Verification items for the finished model (mm, model axes). A direction names the side the tool comes from. Coordinates: 2 decimals unless noted, no trailing zeros. Write each loop counter-clockwise with the first axis right and the second up, starting at its lowest first coordinate (ties: lowest second). Pieces come first, ordered by that corner, then holes. Notation, with made-up numbers: (-15, 71.25) - (32, 71.25) arc R18 cw to (32, 91.25) - close; hole circle Ø6 at (40.25, -4). An arc over 180 degrees is marked (long way). Use one line per item in the form item = value. Start each with the question number.
(1) Sectioned sample at A-A (y = 16). Record the cut outline in (x, z) (3 decimals), and give its area (3 significant figures).
(2) Sectioned sample at B-B (x = 40). Record the cut outline in (y, z).
(3) Material ranges on line 1 (Y direction, x = 3.25, z = 7.75); line 2 (X direction, y = 30.5, z = 9.5); line 3 (Y direction, x = 31.5, z = 28.5), recorded low to high. Write a range as [from, to].
(4) Gauge pin test, flat ends, axial feed: pin 1 Ø12 at (x, z) = (56.5, 8) entering from +Y (3 decimals); pin 2 Ø4 at (x, z) = (74, 4) entering from +Y; pin 3 Ø8 at (y, z) = (30, 25.5) entering from +X. Record the tip position at first contact, or that the pin passes through.
(5) Mould release check, pull along Z, two halves, no side actions. Record for faces 4 (the flat face through (109, 4, 19)), 5 (the cylindrical face through (114.5, 48.1, 28.8)), 6 (the conical face through (3.215, 59.769, 3.142)): released by +Z, released by -Z, zero draft, split by the parting line, or undercut.
(6) Tool access check on faces 1 (the flat face through (27, 83, 16)), 2 (the flat face through (0, 60, 9)), 3 (the cylindrical face through (114.54, 16.24, 18.97)). Record the directions out of +Z, -Z, +X, -X, +Y, -Y that give a thin tool (end or side, any length) a straight path to the whole face; none if there is none.
(7) Sectioned sample at D-D (y = 39). Record the cut outline in (x, z).
(8) Sectioned sample at C-C (z = 0). Record the cut outline in (x, y).
from build123d import *

# Parameters (mm, degrees)
PAD_DEPTH       = 38
POCKET_DEPTH    = 33
SKETCH015_W     = 6
SKETCH015_H     = 6
PAD006_DEPTH    = 15.5
SKETCH018_W     = 36
SKETCH018_H     = 36
PAD008_DEPTH    = 3.5
POCKET008_DEPTH = 8
SKETCH025_R     = 1.7
HOLE_DEPTH      = 12
HOLE_TIPS_R     = 1.7
SKETCH026_R     = 1.7
HOLE003_DEPTH   = 25
HOLE003_TIPS_R  = 1.7
POCKET009_DEPTH = 1


with BuildPart() as part:
    # Sketch → Pad (new body)
    with BuildSketch(Plane.XY):
        Polygon((-8, -2), (117, -2), (117, 98), (82, 98), (62, 83), (-8, 83), align=None)
    extrude(amount=PAD_DEPTH)

    # Sketch001 (on Face8 of Pad) → Pocket (cut)
    with BuildSketch(Plane.XY.offset(38)):
        Polygon((-3, 75), (-3, 6), (0, 6), (0, 3), (109, 3), (109, 6), (112, 6), (112, 90), (109, 90), (109, 93), (83, 93), (63, 78), (0, 78), (0, 75), align=None)
    extrude(amount=-POCKET_DEPTH, mode=Mode.SUBTRACT)

    # Sketch015 → Pad006 (join)
    with BuildSketch(Plane.XY.offset(3)):
        with Locations((3, 60)):
            Rectangle(SKETCH015_W, SKETCH015_H)
        with Locations((87, 60)):
            Rectangle(SKETCH015_W, SKETCH015_H)
        with Locations((3, 6)):
            Rectangle(SKETCH015_W, SKETCH015_H)
        with Locations((87, 6)):
            Rectangle(SKETCH015_W, SKETCH015_H)
    extrude(amount=PAD006_DEPTH)

    # Sketch018 → Pad008 (join)
    with BuildSketch(Plane.XY.offset(3)):
        with Locations((41, 41)):
            Rectangle(SKETCH018_W, SKETCH018_H)
    extrude(amount=PAD008_DEPTH)

    # Sketch014 → Pocket008 (cut)
    with BuildSketch(Plane.YZ.offset(117)):
        with BuildLine():
            ThreePointArc((19.25908, 9.405), (16, 21.475), (12.74092, 9.405))
            Line((12.74092, 9.405), (19.25908, 9.405))
        make_face()
        with BuildLine():
            ThreePointArc((83.25908, 9.405), (80, 21.475), (76.74092, 9.405))
            Line((76.74092, 9.405), (83.25908, 9.405))
        make_face()
        with BuildLine():
            ThreePointArc((69.25908, 22.405), (66, 34.475), (62.74092, 22.405))
            Line((62.74092, 22.405), (69.25908, 22.405))
        make_face()
        with BuildLine():
            ThreePointArc((33.25908, 22.405), (30, 34.475), (26.74092, 22.405))
            Line((26.74092, 22.405), (33.25908, 22.405))
        make_face()
        with BuildLine():
            ThreePointArc((49.746425, 25.2), (48, 31.3), (46.253575, 25.2))
            Line((49.746425, 25.2), (46.253575, 25.2))
        make_face()
        with BuildLine():
            ThreePointArc((42.65, 12.069556), (48, 8.9), (53.35, 12.069556))
            Line((53.35, 17.930444), (53.35, 12.069556))
            ThreePointArc((53.35, 17.930444), (48, 21.1), (42.65, 17.930444))
            Line((42.65, 17.930444), (42.65, 12.069556))
        make_face()
    extrude(amount=-POCKET008_DEPTH, mode=Mode.SUBTRACT)

    # Sketch025 (on Face41 of Pocket008) → Hole (cut)
    with BuildSketch(Plane.XY.offset(18.5)):
        with Locations((3.25, 59.5)):
            Circle(SKETCH025_R)
        with Locations((3.25, 6.5)):
            Circle(SKETCH025_R)
        with Locations((86.75, 6.5)):
            Circle(SKETCH025_R)
        with Locations((86.75, 59.5)):
            Circle(SKETCH025_R)
    extrude(amount=-HOLE_DEPTH, mode=Mode.SUBTRACT)

    # Hole tips → Hole tip 1 section 0
    with BuildSketch(Plane.XY.offset(6.5), mode=Mode.PRIVATE) as hole_tip_1_s0:
        with Locations((3.25, 59.5)):
            Circle(HOLE_TIPS_R)
    loft([hole_tip_1_s0.sketch, Vertex(3.25, 59.5, 5.478537)], mode=Mode.SUBTRACT)

    # Hole tips → Hole tip 2 section 0
    with BuildSketch(Plane.XY.offset(6.5), mode=Mode.PRIVATE) as hole_tip_2_s0:
        with Locations((3.25, 6.5)):
            Circle(HOLE_TIPS_R)
    loft([hole_tip_2_s0.sketch, Vertex(3.25, 6.5, 5.478537)], mode=Mode.SUBTRACT)

    # Hole tips → Hole tip 3 section 0
    with BuildSketch(Plane.XY.offset(6.5), mode=Mode.PRIVATE) as hole_tip_3_s0:
        with Locations((86.75, 6.5)):
            Circle(HOLE_TIPS_R)
    loft([hole_tip_3_s0.sketch, Vertex(86.75, 6.5, 5.478537)], mode=Mode.SUBTRACT)

    # Hole tips → Hole tip 4 section 0
    with BuildSketch(Plane.XY.offset(6.5), mode=Mode.PRIVATE) as hole_tip_4_s0:
        with Locations((86.75, 59.5)):
            Circle(HOLE_TIPS_R)
    loft([hole_tip_4_s0.sketch, Vertex(86.75, 59.5, 5.478537)], mode=Mode.SUBTRACT)

    # Sketch026 (on Face5 of Hole) → Hole003 (cut)
    with BuildSketch(Plane.XY.offset(38)):
        with Locations((-4, 79)):
            Circle(SKETCH026_R)
        with Locations((113, 94)):
            Circle(SKETCH026_R)
        with Locations((113, 2)):
            Circle(SKETCH026_R)
        with Locations((-4, 2)):
            Circle(SKETCH026_R)
    extrude(amount=-HOLE003_DEPTH, mode=Mode.SUBTRACT)

    # Hole003 tips → Hole003 tip 1 section 0
    with BuildSketch(Plane.XY.offset(13), mode=Mode.PRIVATE) as hole003_tip_1_s0:
        with Locations((-4, 79)):
            Circle(HOLE003_TIPS_R)
    loft([hole003_tip_1_s0.sketch, Vertex(-4, 79, 11.978537)], mode=Mode.SUBTRACT)

    # Hole003 tips → Hole003 tip 2 section 0
    with BuildSketch(Plane.XY.offset(13), mode=Mode.PRIVATE) as hole003_tip_2_s0:
        with Locations((113, 94)):
            Circle(HOLE003_TIPS_R)
    loft([hole003_tip_2_s0.sketch, Vertex(113, 94, 11.978537)], mode=Mode.SUBTRACT)

    # Hole003 tips → Hole003 tip 3 section 0
    with BuildSketch(Plane.XY.offset(13), mode=Mode.PRIVATE) as hole003_tip_3_s0:
        with Locations((113, 2)):
            Circle(HOLE003_TIPS_R)
    loft([hole003_tip_3_s0.sketch, Vertex(113, 2, 11.978537)], mode=Mode.SUBTRACT)

    # Hole003 tips → Hole003 tip 4 section 0
    with BuildSketch(Plane.XY.offset(13), mode=Mode.PRIVATE) as hole003_tip_4_s0:
        with Locations((-4, 2)):
            Circle(HOLE003_TIPS_R)
    loft([hole003_tip_4_s0.sketch, Vertex(-4, 2, 11.978537)], mode=Mode.SUBTRACT)

    # Sketch027 (on Face5 of Hole003) → Pocket009 (cut)
    with BuildSketch(Plane.XY.offset(38)):
        with BuildLine():
            ThreePointArc((-4, 81.5), (-5.767767, 80.767767), (-6.5, 79))
            Line((-6.5, 79), (-6.5, 2))
            ThreePointArc((-6.5, 2), (-5.767767, 0.232233), (-4, -0.5))
            Line((-4, -0.5), (113, -0.5))
            ThreePointArc((113, -0.5), (114.767767, 0.232233), (115.5, 2))
            Line((115.5, 2), (115.5, 94))
            ThreePointArc((115.5, 94), (114.767767, 95.767767), (113, 96.5))
            Line((113, 96.5), (82, 96.5))
            Line((82, 96.5), (62, 81.5))
            Line((62, 81.5), (-4, 81.5))
        make_face()
        with BuildLine():
            ThreePointArc((113.5, 4.44949), (111.232233, 3.767767), (110.55051, 1.5))
            Line((110.55051, 1.5), (-1.55051, 1.5))
            ThreePointArc((-1.55051, 1.5), (-2.232233, 3.767767), (-4.5, 4.44949))
            Line((-4.5, 4.44949), (-4.5, 76.55051))
            ThreePointArc((-4.5, 76.55051), (-2.232233, 77.232233), (-1.55051, 79.5))
            Line((-1.55051, 79.5), (62.44949, 79.5))
            Line((62.44949, 79.5), (82.55051, 94.5))
            Line((82.55051, 94.5), (110.55051, 94.5))
            ThreePointArc((110.55051, 94.5), (111.232233, 92.232233), (113.5, 91.55051))
            Line((113.5, 91.55051), (113.5, 4.44949))
        make_face(mode=Mode.SUBTRACT)
    extrude(amount=-POCKET009_DEPTH, mode=Mode.SUBTRACT)


with BuildPart() as part_1:
    # Body placement: moved
    add(part.part.moved(Location((0, 0, -2.5))))


solid = part_1.part
Answers below:
q1.outline = (-8, -2.5) - (117, -2.5) - (117, 6.905) - (112, 6.905) - (112, 2.5) - (-3, 2.5) - (-3, 35.5) - (-4.5, 35.5) - (-4.5, 34.5) - (-6.5, 34.5) - (-6.5, 35.5) - (-8, 35.5) - close; (112, 18.975) - (117, 18.975) - (117, 35.5) - (115.5, 35.5) - (115.5, 34.5) - (113.5, 34.5) - (113.5, 35.5) - (112, 35.5) - close
q1.area = 891 mm2
q2.outline = (-2, -2.5) - (83, -2.5) - (83, 35.5) - (81.5, 35.5) - (81.5, 34.5) - (79.5, 34.5) - (79.5, 35.5) - (78, 35.5) - (78, 2.5) - (59, 2.5) - (59, 4) - (23, 4) - (23, 2.5) - (3, 2.5) - (3, 35.5) - (1.5, 35.5) - (1.5, 34.5) - (-0.5, 34.5) - (-0.5, 35.5) - (-2, 35.5) - close
q3.line_1 = [-2, 4.8], [8.2, 9], [57, 57.8], [61.2, 63], [78, 83]
q3.line_2 = [-8, -3], [112, 117]
q3.line_3 = [-2, 3], [78, 83]
q4.pin_1 = 83.375
q4.pin_2 = 93.5
q4.pin_3 = -3
q5.face_4 = zero draft
q5.face_5 = undercut
q5.face_6 = released by +Z
q6.face_1 = +Z, -Z, -X, +Y
q6.face_2 = +Z
q6.face_3 = +X
q7.outline = (-8, -2.5) - (117, -2.5) - (117, 35.5) - (115.5, 35.5) - (115.5, 34.5) - (113.5, 34.5) - (113.5, 35.5) - (112, 35.5) - (112, 2.5) - (59, 2.5) - (59, 4) - (23, 4) - (23, 2.5) - (-3, 2.5) - (-3, 35.5) - (-4.5, 35.5) - (-4.5, 34.5) - (-6.5, 34.5) - (-6.5, 35.5) - (-8, 35.5) - close
q8.outline = (-8, -2) - (117, -2) - (117, 98) - (82, 98) - (62, 83) - (-8, 83) - close
